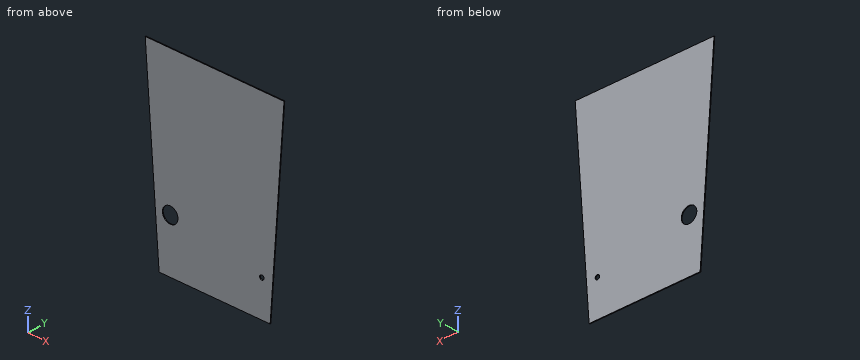
from build123d import *

# Parameters (mm, degrees)
F1_DEPTH = 1.5
F3_D     = 28
F4_D     = 8


with BuildPart() as f1:
    # F0 (on Front) → F1 (new body)
    with BuildSketch(Plane.XZ):
        Polygon((125.04598, 74.155715), (0.04598, 74.155715), (0.04598, -275.844285), (100.04598, -275.844285), align=None)
        Polygon((0.04598, -275.844285), (0.04598, 74.155715), (-124.95402, 74.155715), (-99.95402, -275.844285), align=None)
    extrude(amount=F1_DEPTH)

    # F3 (through all)
    with Locations(Plane.XZ.offset(1.5)):
        with Locations((-79.95402, -180.844285)):
            Hole(F3_D / 2)

    # F4 (through all)
    with Locations(Plane.XZ.offset(1.5)):
        with Locations((85.04598, -210.844285)):
            Hole(F4_D / 2)


solid = f1.part
Here's how the part is built. I have some questions about the finished solid (model axes, mm). Coordinates: 2 decimals unless noted, no trailing zeros. Write each loop counter-clockwise with the first axis right and the second up, starting at its lowest first coordinate (ties: lowest second). Pieces come first, ordered by that corner, then holes.
1) If we section it at A-A (y = -1.2): List the corners of the cut face in (x, z) for me, plus the area to 3 significant figures.
Filled in:
outline: (-124.95, 74.16) - (-99.95, -275.84) - (100.05, -275.84) - (125.05, 74.16) - close; hole circle Ø28 at (-79.95, -180.84); hole circle Ø8 at (85.05, -210.84)
area: 78,100 mm2
2) If we section it at C-C (x = -109): List the corners of the cut face in (y, z) for me.
Filled in:
outline: (-1.5, -149.2) - (0, -149.2) - (0, 74.16) - (-1.5, 74.16) - close
3) If we section it at B-B (z = -131.5): List the corners of the cut face in (x, y) for me.
Filled in:
outline: (-110.26, -1.5) - (110.36, -1.5) - (110.36, 0) - (-110.26, 0) - close
4) If I drill on line 1 (X direction, y = -0.55, z = -172); line 2 (Z direction, x = -85, y = -1.05); line 3 (X direction, y = -0.6, z = -188), over which ranges is the centre line in solid material (lowest first)?
Filled in:
line 1: x = -107.37 to -90.81, -69.1 to 107.46
line 2: z = -275.84 to -193.9, -167.79 to 74.16
line 3: x = -106.23 to -91.99, -67.92 to 106.32
